Can you work these out from the drawing? Everything is in mm from the part's minimum corner. A direction names the side the tool comes from. Coordinates: 2 decimals unless noted, no trailing zeros. Order: outer loops, then holes, each group sorted by start corner. A loop starts at its lowest first (then second) coordinate and runs counter-clockwise, first axis right, second up. Notation, with made-up numbers: (-32, 57) -> (11, 57) arc R31 ccw to (11, 95) -> close; hole circle Ø2 at (-0.5, 89.25). An arc over 180 degrees is marked (long way). Put each result on its own line as item: value. Start each with the question number.
Q1. Please list where these lines run through material, in increasing order: line 1 along X through (y, z) = (11.75, 12.7); line 2 along Y through (x, z) = (15.5, 20.5); line 3 along X through (y, z) = (12.75, 15).
Q2. If we section it at C-C (y = 2.75): Please give me the cut outline in (x, z).
Q3. If we section it at A-A (z = 12.7): Please give me the cut outline in (x, y), and give its area (3 significant figures).
Q4. If we section it at D-D (x = 20.95): Please give me the cut outline in (y, z) (1 decimal).
Q5. For the marked faces 1 and 2, which set-ups out of +Z, -Z, +X, -X, +Y, -Y let a thin tool reach every point of the face, with its end or its side?
Q6. Will these pins go through, and if not, where does the flat tip stop? pin 1 (3 mm diameter, centred on y = 3.5, z = 22.5, fed in from +X); pin 2 (5 mm diameter, centred on x = 14, y = 12, fed in from -Z); pin 3 (1.5 mm diameter, centred on x = 17, y = 15, fed in from -Z).
Q7. We'd pull the mould along X, two halves only. Please class the marked faces 3, 4 and 5: +X half, -X half, draft (parallel to the pull), parting line (faces both ways), or undercut.
Q8. If we section it at B-B (x = 12.7): Please give me the cut outline in (y, z), and give its area (3 significant figures).
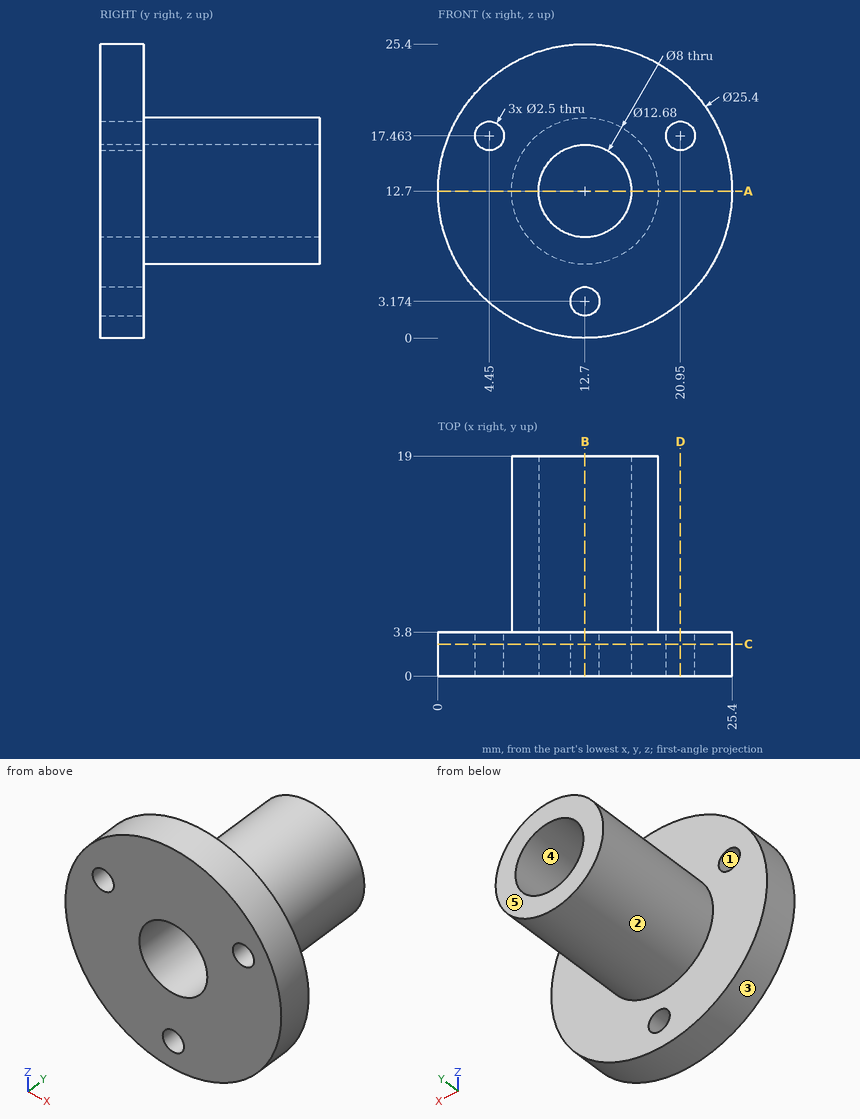
The answers:
1. line 1: 6.36 to 8.7, 16.7 to 19.04
1. line 2: 0 to 3.8
1. line 3: 6.79 to 9.43, 15.97 to 18.61
2. outline: circle Ø25.4 at (12.7, 12.7); hole circle Ø2.5 at (4.45, 17.46); hole circle Ø8 at (12.7, 12.7); hole circle Ø2.5 at (12.7, 3.17); hole circle Ø2.5 at (20.95, 17.46)
3. outline: (0, 0) -> (8.7, 0) -> (8.7, 19) -> (6.36, 19) -> (6.36, 3.8) -> (0, 3.8) -> close; (16.7, 0) -> (25.4, 0) -> (25.4, 3.8) -> (19.04, 3.8) -> (19.04, 19) -> (16.7, 19) -> close
3. area: 137 mm^2
4. outline: (0, 3) -> (3.8, 3) -> (3.8, 16.2) -> (0, 16.2) -> close; (0, 18.7) -> (3.8, 18.7) -> (3.8, 22.4) -> (0, 22.4) -> close
5. face 1: +Y, -Y
5. face 2: +Y
6. pin 1: x = 22.31
6. pin 2: z = 6.36
6. pin 3: z = 7.45
7. face 3: parting line
7. face 4: undercut
7. face 5: draft
8. outline: (0, 0) -> (3.8, 0) -> (3.8, 1.92) -> (0, 1.92) -> close; (0, 4.42) -> (3.8, 4.42) -> (3.8, 6.36) -> (19, 6.36) -> (19, 8.7) -> (0, 8.7) -> close; (0, 16.7) -> (19, 16.7) -> (19, 19.04) -> (3.8, 19.04) -> (3.8, 25.4) -> (0, 25.4) -> close
8. area: 128 mm^2
